Could you check a few things on this model? Use its own coordinates, in mm. A direction names the side the tool comes from. Round coordinates to 2 decimals unless told otherwise and drop trailing zeros. Write each loop counter-clockwise with the first axis right and the second up, starting at its lowest first coordinate (ties: lowest second). Pieces come first, ordered by that corner, then holes. Notation, with made-up numbers: (-8, 7.25) - (27, 7.25) arc R25 ccw to (27, 45.25) - close; hole circle Ø3 at (55, 67). An arc over 180 degrees is marked (long way). Write each question's results on one line, items separated by ' | '. Start each with the question number.
(1) Please list where these lines run through material, in increasing order: line 1 (X direction, y = 4.5, z = 0); line 2 (Z direction, x = 4.5, y = 34.5); line 3 (X direction, y = 4.5, z = -25.4). Write a range as [from, to].
(2) Imagine slicing it at D-D on x = 25.4. Write out the boundary of the cut face in (y, z).
(3) Imagine slicing it at B-B on y = 13.5. State how many separate pieces and enclosed holes the cut face has, then the cut area to 3 significant figures.
(4) Imagine slicing it at C-C on z = 0. Write out the boundary of the cut face in (x, y), then the cut area to 3 significant figures.
(5) On a 3-axis mill with a long thin cutter (end or side, diameter ignored), from which of +Z, -Z, +X, -X, +Y, -Y can I reach the whole of each face in a straight line? I mean faces 4 (the flat face through (-9.525, 23, 45)), 5 (the flat face through (-45, 23, 9.525)), 6 (the flat face through (9.525, 23, 45)), 7 (the flat face through (0, 23, -38.481)). Say none if no direction works.
(6) Thinking about a two-plate mould opening in Z: for faces 1 (the cylindrical face through (-13.77, 3.13, 61.99)), 2 (the cylindrical face through (23.1, 3.1, 27.2)), 3 (the flat face through (38.621, 22, 0)), which applies, +Z half, -Z half, draft (parallel to the pull), parting line (faces both ways), or undercut?
(7) Imagine slicing it at A-A on x = 0. Write out the boundary of the cut face in (y, z), then the cut area to 3 significant figures.
(8) For P1, Ø12.5, axis at x = 0, z = 0, coming from the +Y side; P2, Ø11, axis at y = 20, z = 2, coming from the +X side; P3, Ø8.5, axis at x = -43.5, y = 24, coming from the +Z side (3 decimals), each with a flat end and sliding along its axis, tell me the tip position at first contact or that it passes through.
```python
from build123d import *

# Parameters (mm, degrees)
SKETCH2_R           = 63.5
SKETCH2_R_2         = 2.921
SKETCH2_R_3         = 4.826
BOSS_EXTRUDE2_DEPTH = 6.35
SKETCH3_W           = 19.05
SKETCH3_H           = 12.7
SKETCH3_W_2         = 12.7
SKETCH3_H_2         = 19.05
BOSS_EXTRUDE3_DEPTH = 31.75
FILLET1_R           = 2.54


with BuildPart() as part:
    # Sketch2 → Boss-Extrude2 (new body)
    with BuildSketch(Plane(origin=(0, 0, 0), x_dir=(1, 0, 0), z_dir=(0, 1, 0))):
        Circle(SKETCH2_R)
        with Locations((-25.4, 25.4)):
            Circle(SKETCH2_R_2, mode=Mode.SUBTRACT)
        with Locations((25.4, 25.4)):
            Circle(SKETCH2_R_2, mode=Mode.SUBTRACT)
        with Locations((25.4, -25.4)):
            Circle(SKETCH2_R_2, mode=Mode.SUBTRACT)
        with Locations((-25.4, -25.4)):
            Circle(SKETCH2_R_2, mode=Mode.SUBTRACT)
        Circle(SKETCH2_R_3, mode=Mode.SUBTRACT)
    extrude(amount=BOSS_EXTRUDE2_DEPTH)

    # Sketch3 → Boss-Extrude3 (add)
    with BuildSketch(Plane(origin=(0, 6.35, 0), x_dir=(1, 0, 0), z_dir=(0, 1, 0))):
        with Locations((0, 44.831)):
            Rectangle(SKETCH3_W, SKETCH3_H)
        with Locations((0, -44.831)):
            Rectangle(SKETCH3_W, SKETCH3_H)
        with Locations((-44.971451378, 0)):
            Rectangle(SKETCH3_W_2, SKETCH3_H_2)
        with Locations((44.971451378, 0)):
            Rectangle(SKETCH3_W_2, SKETCH3_H_2)
    extrude(amount=BOSS_EXTRUDE3_DEPTH)

    # Fillet1
    fillet1_edges = [part.edges().sort_by_distance(p)[0] for p in [
        (9.525, 6.35, -44.831),
        (9.525, 22.225, -38.481),
        (0, 6.35, -51.181),
        (9.525, 22.225, -51.181),
        (-9.525, 6.35, -44.831),
        (-9.525, 22.225, -51.181),
        (0, 6.35, -38.481),
        (-9.525, 22.225, -38.481),
        (-9.525, 6.35, 44.831),
        (-9.525, 22.225, 38.481),
        (0, 6.35, 51.181),
        (-9.525, 22.225, 51.181),
        (9.525, 6.35, 44.831),
        (9.525, 22.225, 51.181),
        (0, 6.35, 38.481),
        (9.525, 22.225, 38.481),
        (0, 38.1, 38.481),
        (-38.621451378, 6.35, 0),
        (-38.621451378, 22.225, 9.525),
        (-44.971451378, 6.35, -9.525),
        (-38.621451378, 22.225, -9.525),
        (-51.321451378, 6.35, 0),
        (-51.321451378, 22.225, -9.525),
        (-44.971451378, 6.35, 9.525),
        (-51.321451378, 22.225, 9.525),
        (44.971451378, 6.35, -9.525),
        (51.321451378, 22.225, -9.525),
        (38.621451378, 6.35, 0),
        (38.621451378, 22.225, -9.525),
        (44.971451378, 6.35, 9.525),
        (38.621451378, 22.225, 9.525),
        (51.321451378, 6.35, 0),
        (51.321451378, 22.225, 9.525),
        (38.621451378, 38.1, 0),
    ]]
    fillet(fillet1_edges, radius=FILLET1_R)


solid = part.part
```
Response:
1) line 1: [-63.5, -4.83], [4.83, 63.5] | line 2: [-51.18, -38.48], [38.48, 51.18] | line 3: [-58.2, -28.32], [-22.48, 22.48], [28.32, 58.2]
2) outline: (0, -58.2) - (6.35, -58.2) - (6.35, -28.32) - (0, -28.32) - close; (0, -22.48) - (6.35, -22.48) - (6.35, 22.48) - (0, 22.48) - close; (0, 28.32) - (6.35, 28.32) - (6.35, 58.2) - (0, 58.2) - close
3) separate pieces: 4 | enclosed holes: 0 | area: 946 mm²
4) outline: (-63.5, 0) - (-4.83, 0) - (-4.83, 6.35) - (-36.08, 6.35) arc R2.54 cw to (-38.62, 8.89) - (-38.62, 38.1) - (-51.32, 38.1) - (-51.32, 8.89) arc R2.54 cw to (-53.86, 6.35) - (-63.5, 6.35) - close; (4.83, 0) - (63.5, 0) - (63.5, 6.35) - (53.86, 6.35) arc R2.54 cw to (51.32, 8.89) - (51.32, 38.1) - (41.16, 38.1) arc R2.54 ccw to (38.62, 35.56) - (38.62, 8.89) arc R2.54 cw to (36.08, 6.35) - (4.83, 6.35) - close | area: 1,560 mm²
5) face 4: +Z, -Z, -X, +Y | face 5: +Z, +X, -X, +Y | face 6: +Z, -Z, +X, +Y | face 7: +X, -X, +Y
6) face 1: parting line | face 2: undercut | face 3: draft
7) outline: (0, -63.5) - (6.35, -63.5) - (6.35, -53.72) arc R2.54 cw to (8.89, -51.18) - (38.1, -51.18) - (38.1, -38.48) - (8.89, -38.48) arc R2.54 cw to (6.35, -35.94) - (6.35, -4.83) - (0, -4.83) - close; (0, 4.83) - (6.35, 4.83) - (6.35, 35.94) arc R2.54 cw to (8.89, 38.48) - (35.56, 38.48) arc R2.54 ccw to (38.1, 41.02) - (38.1, 51.18) - (8.89, 51.18) arc R2.54 cw to (6.35, 53.72) - (6.35, 63.5) - (0, 63.5) - close | area: 1,560 mm²
8) P1: y = 6.35 | P2: x = 51.32 | P3: z = 9.525
